```python
from build123d import *

# Parameters (mm, degrees)
CHAMFER_1_SIZE      = 1
CHAMFER_2_SIZE      = 2
CUT_EXTRUDE_START   = 17
SKETCH_2_OUTSIDE_W  = 110.37
SKETCH_2_OUTSIDE_H  = 110.37
SKETCH_2_OUTSIDE_R  = 11.95
CUT_EXTRUDE_1_DEPTH = 1.3
CUT_EXTRUDE_2_DEPTH = 130
FILLET_1_R          = 130
CUT_EXTRUDE_START_2 = 7
CUT_EXTRUDE_3_DEPTH = 358.341529437
CUT_EXTRUDE_START_3 = 12.5
CUT_EXTRUDE_4_DEPTH = 352.841529437


with BuildPart() as part:
    # 草图1 → 旋转1 (revolve)
    with BuildSketch(Plane.XY):
        Polygon((0, 0), (0, 17.5), (100, 17.5), (100, 12.5), (124.5, 12.5), (124.5, 11), (225.5, 11), (225.5, 10.5), (363.5, 10.5), (363.5, 0), align=None)
    revolve(axis=Axis((363.5, 0, 0), (-1, 0, 0)))

    # 倒角1
    chamfer_1_edges = [part.edges().sort_by_distance(p)[0] for p in [
        (0, -17.5, 0),
    ]]
    chamfer(chamfer_1_edges, length=CHAMFER_1_SIZE)

    # 倒角2
    chamfer_2_edges = [part.edges().sort_by_distance(p)[0] for p in [
        (363.5, -10.5, 0),
    ]]
    chamfer(chamfer_2_edges, length=CHAMFER_2_SIZE)

    # 草图2 outside → 切除-拉伸1 (cut)
    with BuildSketch(Plane(origin=(100, 0, 0), x_dir=(0, 0, -1), z_dir=(1, 0, 0)).offset(CUT_EXTRUDE_START)):
        Rectangle(SKETCH_2_OUTSIDE_W, SKETCH_2_OUTSIDE_H)
        with Locations(Location((0, 0, 0), (0, 0, 90))):
            Circle(SKETCH_2_OUTSIDE_R, mode=Mode.SUBTRACT)
    extrude(amount=CUT_EXTRUDE_1_DEPTH, mode=Mode.SUBTRACT)

    # 草图3 → 切除-拉伸2 (cut)
    with BuildSketch(Plane(origin=(363.5, 0, 0), x_dir=(0, 0, -1), z_dir=(1, 0, 0))):
        with BuildLine():
            Line((-10.062305899, 3), (-7.95298686, 3))
            ThreePointArc((-7.95298686, 3), (-6.01040764, 6.01040764), (-3, 7.95298686))
            Line((-3, 7.95298686), (-3, 10.062305899))
            ThreePointArc((-3, 10.062305899), (-7.424621202, 7.424621202), (-10.062305899, 3))
        make_face()
        with BuildLine():
            Line((3, 10.062305899), (3, 7.95298686))
            ThreePointArc((3, 7.95298686), (6.01040764, 6.01040764), (7.95298686, 3))
            Line((7.95298686, 3), (10.062305899, 3))
            ThreePointArc((10.062305899, 3), (7.424621202, 7.424621202), (3, 10.062305899))
        make_face()
        with BuildLine():
            ThreePointArc((7.95298686, -3), (6.01040764, -6.01040764), (3, -7.95298686))
            Line((3, -7.95298686), (3, -10.062305899))
            ThreePointArc((3, -10.062305899), (7.424621202, -7.424621202), (10.062305899, -3))
            Line((10.062305899, -3), (7.95298686, -3))
        make_face()
        with BuildLine():
            ThreePointArc((-10.062305899, -3), (-7.424621202, -7.424621202), (-3, -10.062305899))
            Line((-3, -10.062305899), (-3, -7.95298686))
            ThreePointArc((-3, -7.95298686), (-6.01040764, -6.01040764), (-7.95298686, -3))
            Line((-7.95298686, -3), (-10.062305899, -3))
        make_face()
    extrude(amount=-CUT_EXTRUDE_2_DEPTH, mode=Mode.SUBTRACT)

    # 圆角1
    # the kernel refuses this fillet: 130 mm, written as the material it adds along each edge
    with BuildSketch(Plane(origin=(233.5, 0, 0), x_dir=(0, 0.7048818539423689, -0.7093247295722663), z_dir=(0, 0.7093247295722663, 0.7048818539423689))) as fillet_1_piece_1:
        with BuildLine():
            CenterArc((138.5, -22.715633383), FILLET_1_R, 169.936725557, 10.063274443)
            Line((10.5, 0), (8.5, 0))
            Line((8.5, 0), (8.5, -22.715633383))
        make_face()
    revolve(axis=Axis((233.5, 0, 0), (-1, 0, 0)), revolution_arc=359.64)
    with BuildSketch(Plane(origin=(233.5, 0, 0), x_dir=(0, 0.7093247295722621, 0.7048818539423733), z_dir=(0, -0.7048818539423733, 0.7093247295722621))) as fillet_1_piece_2:
        with BuildLine():
            CenterArc((138.5, -22.715633383), FILLET_1_R, 169.936725557, 10.063274443)
            Line((10.5, 0), (8.5, 0))
            Line((8.5, 0), (8.5, -22.715633383))
        make_face()
    revolve(axis=Axis((233.5, 0, 0), (-1, 0, 0)), revolution_arc=359.64)
    with BuildSketch(Plane(origin=(233.5, 0, 0), x_dir=(0, -0.7048818539423463, 0.7093247295722888), z_dir=(0, -0.7093247295722888, -0.7048818539423463))) as fillet_1_piece_3:
        with BuildLine():
            CenterArc((138.5, -22.715633383), FILLET_1_R, 169.936725557, 10.063274443)
            Line((10.5, 0), (8.5, 0))
            Line((8.5, 0), (8.5, -22.715633383))
        make_face()
    revolve(axis=Axis((233.5, 0, 0), (-1, 0, 0)), revolution_arc=359.64)
    with BuildSketch(Plane(origin=(233.5, 0, 0), x_dir=(0, -0.7093247295722879, -0.7048818539423474), z_dir=(0, 0.7048818539423474, -0.7093247295722879))) as fillet_1_piece_4:
        with BuildLine():
            CenterArc((138.5, -22.715633383), FILLET_1_R, 169.936725557, 10.063274443)
            Line((10.5, 0), (8.5, 0))
            Line((8.5, 0), (8.5, -22.715633383))
        make_face()
    revolve(axis=Axis((233.5, 0, 0), (-1, 0, 0)), revolution_arc=359.64)

    # 草图4 → 切除-拉伸3 (cut, through all)
    with BuildSketch(Plane.XY.offset(CUT_EXTRUDE_START_2)):
        with BuildLine():
            Line((165, 3), (209, 3))
            ThreePointArc((209, 3), (212, 0), (209, -3))
            Line((209, -3), (165, -3))
            ThreePointArc((165, -3), (162, 0), (165, 3))
        make_face()
    extrude(amount=CUT_EXTRUDE_3_DEPTH, mode=Mode.SUBTRACT)

    # 草图5 → 切除-拉伸4 (cut, through all)
    with BuildSketch(Plane.XY.offset(CUT_EXTRUDE_START_3)):
        with BuildLine():
            Line((10, 5), (40, 5))
            ThreePointArc((40, 5), (45, 0), (40, -5))
            Line((40, -5), (10, -5))
            ThreePointArc((10, -5), (5, 0), (10, 5))
        make_face()
    extrude(amount=CUT_EXTRUDE_4_DEPTH, mode=Mode.SUBTRACT)


solid = part.part
```
Can you work these out from the model? Positions are in its coordinate system, mm. A direction names the side the tool comes from. Round coordinates to 2 decimals unless told otherwise and drop trailing zeros. Loops run counter-clockwise (first coordinate to the right, second up) from the corner with the lowest first, then second, coordinate; pieces in that order, holes last.
Item 1: Will these pins go through, and if not, where does the flat tip stop? pin 1 Ø1.1 at (x, y) = (284.5, -9.5) entering from -Z; pin 2 Ø1.8 at (x, z) = (194.5, 9) entering from -Y; pin 3 Ø2 at (x, z) = (132.5, 0) entering from +Y.
Item 2: If we mould it in two halves opening along Y, with no side actions, what happens to faces 4 (the flat face through (187, 0, 7)), 5 (the cylindrical face through (175.707, 5.914, -9.275)), 6 (the flat face through (25, 0, 12.5)), 7 (the flat face through (363.5, 0, 0))? For each: +Y half, -Y half, draft (parallel to the pull), parting line (faces both ways), or undercut.
Item 3: Suppose I cut it at A-A, the plane x = 299. Write out the boundary of the cut face in (y, z), then the cut area to 3 significant figures.
Item 4: Which directions (+Z, -Z, +X, -X, +Y, -Y) give clear straight access to the entire face, cutting with the end or side of a thin tool? Please do faces 1 (the flat face through (225.5, 10, 4)), 2 (the cylindrical face through (117.641, -1.556, 11.848)), 3 (the cylindrical face through (51.193, 9.408, -14.756)).
Item 5: Please list where these lines run through material, in increasing order: L1, parallel to X at y = 12, z = 3; L2, parallel to X at y = -15, z = 5.5; L3, parallel to X at y = 8.5, z = -0.5.
Item 6: Suppose I cut it at B-B, the plane z = 0. Write out the boundary of the cut face in (x, y).
Item 7: Suppose I cut it at C-C, the plane x = 27. Write out the boundary of the cut face in (y, z), then the cut area to 3 significant figures.
Reported:
1. pin 1: stops at z = -3
1. pin 2: stops at y = -7.44
1. pin 3: stops at y = 11
2. face 4: undercut
2. face 5: parting line
2. face 6: undercut
2. face 7: draft
3. outline: (-10.06, -3) - (-7.95, -3) arc R8.5 ccw to (-3, -7.95) - (-3, -10.06) arc R10.5 ccw to (3, -10.06) - (3, -7.95) arc R8.5 ccw to (7.95, -3) - (10.06, -3) arc R10.5 ccw to (10.06, 3) - (7.95, 3) arc R8.5 ccw to (3, 7.95) - (3, 10.06) arc R10.5 ccw to (-3, 10.06) - (-3, 7.95) arc R8.5 ccw to (-7.95, 3) - (-10.06, 3) arc R10.5 ccw to start
3. area: 276 mm2
4. face 1: +X
4. face 2: none
4. face 3: +X, -X
5. L1: x = 0 to 117, 118.3 to 124.5
5. L2: x = 0 to 100
5. L3: x = 0 to 363.49
6. outline: (0, -16.5) - (1, -17.5) - (100, -17.5) - (100, -12.5) - (117, -12.5) - (117, -11.95) - (118.3, -11.95) - (118.3, -12.5) - (124.5, -12.5) - (124.5, -11) - (225.5, -11) - (225.5, -10.5) - (361.5, -10.5) - (363.5, -8.5) - (363.5, 8.5) - (361.5, 10.5) - (225.5, 10.5) - (225.5, 11) - (124.5, 11) - (124.5, 12.5) - (118.3, 12.5) - (118.3, 11.95) - (117, 11.95) - (117, 12.5) - (100, 12.5) - (100, 17.5) - (1, 17.5) - (0, 16.5) - close
7. outline: (-5, 12.5) - (-5, 16.77) arc R17.5 ccw (long way) to (5, 16.77) - (5, 12.5) - close
7. area: 915 mm2
